The listing builds one solid part. Answer for the finished solid, in the listing's coordinates (mm). Give positions to 0.01 mm unless a question says otherwise; leave off trailing zeros. Order: outer loops, then holes, each group sorted by start corner. A loop starts at its lowest first (then second) coordinate and runs counter-clockwise, first axis right, second up. Notation, with made-up numbers: (-14, 20) - (6, 20) arc R16 cw to (6, 47) - close; hole circle Ø9 at (17.5, 13). An arc over 180 degrees is marked (long way). Answer as a JSON object with one key per item and string values. Group by question number.
Q1. The mould has two halves that part along X. Classify faces 1 (the face through (0, -209, 3)), 2 (the face through (25, 0, 3)), 3 (the face through (50.8, -209, 3)), 4 (the face through (15.53, -22.18, 3.2)): released by +X, released by -X, zero draft, split by the parting line, or undercut.
Q2. Given pin 1 (8.5 mm diameter, centred on x = 19.04, y = -25.4, fed in from -Z), flat-ended and moving along its own axis, determine where the tip first touches the part or whether it passes through.
Q3. A cutting plane is placed at A-A, the plane x = 38.1. Give the vertices of the cut face in (y, z), and give its area (3 significant figures).
Q4. Consider line 1 (Y direction, x = 38.1, z = 4.5); line 2 (Y direction, x = 12.7, z = 3.25). Determine where each line is inside the solid, lowest interval first.
Q5. A cutting plane is placed at B-B, the plane y = -25.4. Give the vertices of the cut face in (x, z).
from build123d import *

# Parameters (mm, degrees)
SALIENTE_EXTRUIR1_DEPTH = 6.31
CROQUIS3_R              = 4.7625
CORTAR_EXTRUIR1_DEPTH   = 9.525
CROQUIS4_R              = 5
CORTAR_EXTRUIR2_DEPTH   = 9.525


with BuildPart() as part:
    # Croquis2 → Saliente-Extruir1 (new body)
    with BuildSketch(Plane.XY):
        Polygon((0, 0), (50.8, 0), (50.8, -361.29566061), (50.8, -412.09566061), (0, -412.09566061), align=None)
    extrude(amount=SALIENTE_EXTRUIR1_DEPTH)

    # Croquis3 → Cortar-Extruir1 (cut)
    with BuildSketch(Plane.XY.offset(6.31)):
        with Locations((19.04, -25.4)):
            Circle(CROQUIS3_R)
    extrude(amount=-CORTAR_EXTRUIR1_DEPTH, mode=Mode.SUBTRACT)

    # Croquis4 → Cortar-Extruir2 (cut)
    with BuildSketch(Plane.XY.offset(6.31)):
        with Locations((12.7, -373.995660606)):
            Circle(CROQUIS4_R)
        with Locations((38.1, -399.395660606)):
            Circle(CROQUIS4_R)
    extrude(amount=-CORTAR_EXTRUIR2_DEPTH, mode=Mode.SUBTRACT)


solid = part.part
Reply:
{
 "1": {"face 1": "released by -X", "face 2": "zero draft", "face 3": "released by +X", "face 4": "undercut"},
 "2": {"pin 1": "passes through"},
 "3": {"outline": "(-412.1, 0) - (-404.4, 0) - (-404.4, 6.31) - (-412.1, 6.31) - close; (-394.4, 0) - (0, 0) - (0, 6.31) - (-394.4, 6.31) - close", "area": "2,540 mm^2"},
 "4": {"line 1": "y = -412.1 to -404.4, -394.4 to 0", "line 2": "y = -412.1 to -379, -369 to 0"},
 "5": {"outline": "(0, 0) - (14.28, 0) - (14.28, 6.31) - (0, 6.31) - close; (23.8, 0) - (50.8, 0) - (50.8, 6.31) - (23.8, 6.31) - close"}
}
